from build123d import *

# Parameters (mm, degrees)
SKETCH1_W           = 60
SKETCH1_H           = 34
SKETCH1_R           = 1.75
BOSS_EXTRUDE1_DEPTH = 4
SKETCH3_W           = 48
SKETCH3_H           = 34
SKETCH3_R           = 13.5
BOSS_EXTRUDE2_DEPTH = 8
FILLET4_R           = 1
FILLET5_R           = 1


with BuildPart() as part:
    # Sketch1 → Boss-Extrude1 (new body)
    with BuildSketch(Plane(origin=(0, 0, 0), x_dir=(0, 0, -1), z_dir=(1, 0, 0))):
        Rectangle(SKETCH1_W, SKETCH1_H)
        with Locations((-6, 0)):
            Circle(SKETCH1_R, mode=Mode.SUBTRACT)
        with Locations(Location((6, 0, 0), (0, 0, 180))):
            Circle(SKETCH1_R, mode=Mode.SUBTRACT)
    extrude(amount=-BOSS_EXTRUDE1_DEPTH)

    # Sketch3 → Boss-Extrude2 (add)
    with BuildSketch(Plane.XY.offset(30)):
        with Locations((20, 0)):
            Rectangle(SKETCH3_W, SKETCH3_H)
        with Locations((27, 0)):
            Circle(SKETCH3_R, mode=Mode.SUBTRACT)
    boss_extrude2 = extrude(amount=BOSS_EXTRUDE2_DEPTH)

    # Mirror1: Boss-Extrude2 across plane
    add(boss_extrude2.mirror(Plane(origin=(0, 0, 0), x_dir=(1, 0, 0), z_dir=(0, 0, -1))))

    # Fillet4
    fillet4_edges = [part.edges().sort_by_distance(p)[0] for p in [
        (0, 0, 30),
    ]]
    fillet(fillet4_edges, radius=FILLET4_R)

    # Fillet5
    fillet5_edges = [part.edges().sort_by_distance(p)[0] for p in [
        (0, 0, -30),
    ]]
    fillet(fillet5_edges, radius=FILLET5_R)


solid = part.part
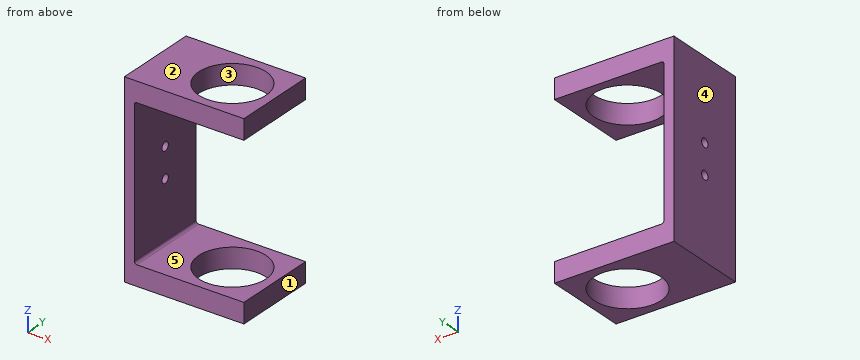
Design review of the part built by this model. Coordinates are the model's own, in mm. Face numbers are marked on the shaded views. A direction names the side the tool comes from. Give positions to 0.01 mm unless a question says otherwise; leave off trailing zeros. Order: outer loops, then holes, each group sorted by start corner. A loop starts at its lowest first (then second) coordinate and runs counter-clockwise, first axis right, second up.
1. Add section C-C, the plane z = -6. State the section outline as (x, y) points.
Solution:
outline: (-4, -17) - (0, -17) - (0, -1.75) - (-4, -1.75) - close; (-4, 1.75) - (0, 1.75) - (0, 17) - (-4, 17) - close
2. Add section D-D, the plane y = 14.5. State the section outline as (x, z) points, then the cut area to 3 significant figures.
Solution:
outline: (-4, -38) - (44, -38) - (44, -30) - (1, -30) arc R1 cw to (0, -29) - (0, 29) arc R1 cw to (1, 30) - (44, 30) - (44, 38) - (-4, 38) - close
area: 1,010 mm2
3. For pin 1 Ø1.5 at (y, z) = (-11, 6) entering from +X; pin 2 Ø17 at (x, y) = (18.5, -8.5) entering from -Z; pin 3 Ø3 at (y, z) = (0, -6) entering from +X, all flat-tipped, find the tip position at first contact; note any pin that passes through.
Solution:
pin 1: stops at x = 0
pin 2: stops at z = -38
pin 3: passes through
4. To check wall thickness, follow L1, parallel to Z at x = 27, y = -15; L2, parallel to Y at x = 27, z = 33.5; L3, parallel to Y at x = -1.8, z = -6. State the ranges of each line that lie inside material, in increasing order.
Solution:
L1: z = -38 to -30, 30 to 38
L2: y = -17 to -13.5, 13.5 to 17
L3: y = -17 to -1.75, 1.75 to 17
5. Tool access review of the marked faces 4 and 5: name each direction out of +Z, -Z, +X, -X, +Y, -Y from which nothing blocks a thin tool from reaching the whole face with its end or side.
Solution:
face 4: +Z, -Z, -X, +Y, -Y
face 5: +X, +Y, -Y
6. Add section A-A, the plane x = 27. State the section outline as (y, z) points.
Solution:
outline: (-17, -38) - (-13.5, -38) - (-13.5, -30) - (-17, -30) - close; (-17, 30) - (-13.5, 30) - (-13.5, 38) - (-17, 38) - close; (13.5, -38) - (17, -38) - (17, -30) - (13.5, -30) - close; (13.5, 30) - (17, 30) - (17, 38) - (13.5, 38) - close
7. Add section B-B, the plane y = 0. State the section outline as (x, z) points, then the cut area to 3 significant figures.
Solution:
outline: (-4, -38) - (13.5, -38) - (13.5, -30) - (1, -30) arc R1 cw to (0, -29) - (0, -7.75) - (-4, -7.75) - close; (-4, -4.25) - (0, -4.25) - (0, 4.25) - (-4, 4.25) - close; (-4, 7.75) - (0, 7.75) - (0, 29) arc R1 cw to (1, 30) - (13.5, 30) - (13.5, 38) - (-4, 38) - close; (40.5, -38) - (44, -38) - (44, -30) - (40.5, -30) - close; (40.5, 30) - (44, 30) - (44, 38) - (40.5, 38) - close
area: 548 mm2
8. Mouldability with a two-part tool opening along X and no side actions: class the marked faces 1, 2 and 3 as +X half, -X half, draft (parallel to the pull), parting line (faces both ways), or undercut.
Solution:
face 1: +X half
face 2: draft
face 3: undercut
